Input: part model. Units: mm. Frame: model coordinates. Coordinates: 2 decimals unless noted, no trailing zeros. Loops run counter-clockwise (first coordinate to the right, second up) from the corner with the lowest first, then second, coordinate; pieces in that order, holes last.
Item 1: Ray query, line 1 along Y through (x, z) = (-0.5, 27); line 2 along X through (y, z) = (-46.5, 7); line 3 along X through (y, z) = (-84, 7). Return the intervals inside material, ascending.
Item 2: Section A-A on z = 15.5. Return loops of the section in (x, y).
Item 3: Contact query for flat-ended pins moving along their axis: P1, Ø5, axis at y = -46.5, z = 20, coming from the +X side; P2, Ø2, axis at y = -24.5, z = 45, coming from the +X side; P3, Ø12, axis at x = -56, z = 10.5, coming from the -Y side. Output: stop coordinate, or through.
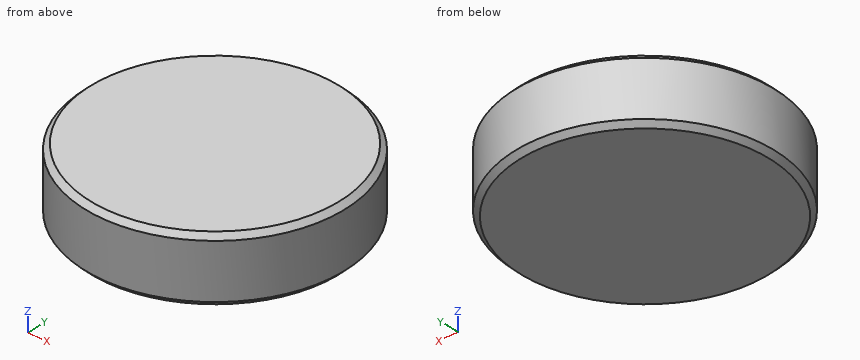
```python
from build123d import *

# Parameters (mm, degrees)
ESQUISSE1_R        = 100
BOSS_EXTRU_1_DEPTH = 50
CHANFREIN1_SIZE    = 4
CHANFREIN2_SIZE    = 4


with BuildPart() as part:
    # Esquisse1 → Boss.-Extru.1 (new body)
    with BuildSketch(Plane.XY):
        Circle(ESQUISSE1_R)
    extrude(amount=BOSS_EXTRU_1_DEPTH)

    # Chanfrein1
    chanfrein1_edges = [part.edges().sort_by_distance(p)[0] for p in [
        (-100, 0, 0),
    ]]
    chamfer(chanfrein1_edges, length=CHANFREIN1_SIZE)

    # Chanfrein2
    chanfrein2_edges = [part.edges().sort_by_distance(p)[0] for p in [
        (-100, 0, 50),
    ]]
    chamfer(chanfrein2_edges, length=CHANFREIN2_SIZE)


solid = part.part
```
Results found:
1. line 1: y = -100 to 100
1. line 2: x = -88.53 to 88.53
1. line 3: x = -54.26 to 54.26
2. outline: circle Ø200 at (0, 0)
3. P1: stops at x = 89.8
3. P2: stops at x = 97.2
3. P3: stops at y = -86.6
